Geometry check sheet. Reference: the model listing, model coordinates, mm. A direction names the side the tool comes from. Coordinates: 2 decimals unless noted, no trailing zeros. Loops run counter-clockwise (first coordinate to the right, second up) from the corner with the lowest first, then second, coordinate; pieces in that order, holes last. Notation, with made-up numbers: M 42,22 L 95,22 A24 ccw 95,48 Z; hole C 17,46 d1. An arc over 180 degrees is marked long. One line per question, with ' | ' between items. Start each with the question number.
from build123d import *

# Parameters (mm, degrees)
ESQUISSE1_R             = 12.5
ESQUISSE1_R_2           = 1.25
ESQUISSE1_R_3           = 2.613961031
DISQUE_O25_DEPTH        = 2.5
ESQUISSE2_R             = 5
ESQUISSE2_R_2           = 2.9
MOYEU_CANNELE_25T_DEPTH = 3.5


with BuildPart() as part:
    # Esquisse1 → Disque O25 (new body)
    with BuildSketch(Plane.XY):
        Circle(ESQUISSE1_R)
        with Locations((5, 0)):
            Circle(ESQUISSE1_R_2, mode=Mode.SUBTRACT)
        with Locations((-5, 0)):
            Circle(ESQUISSE1_R_2, mode=Mode.SUBTRACT)
        with Locations((5, 6.363961031)):
            Circle(ESQUISSE1_R_3, mode=Mode.SUBTRACT)
        with Locations((5, -6.363961031)):
            Circle(ESQUISSE1_R_3, mode=Mode.SUBTRACT)
    extrude(amount=DISQUE_O25_DEPTH)

    # Esquisse2 → Moyeu cannele 25T (add)
    with BuildSketch(Plane.XY):
        Circle(ESQUISSE2_R)
        Circle(ESQUISSE2_R_2, mode=Mode.SUBTRACT)
    extrude(amount=-MOYEU_CANNELE_25T_DEPTH)


solid = part.part
1. Tool access check on faces 1 (the cylindrical face through (-6.25, 0.05, 1.23)), 2 (the flat face through (0, 0, 0)), 3 (the cylindrical face through (2.39, 6.48, 1.23)). Record the directions out of +Z, -Z, +X, -X, +Y, -Y that give a thin tool (end or side, any length) a straight path to the whole face; none if there is none.
2. Sectioned sample at B-B (y = -5.75). Record the cut outline in (x, z).
3. Thickness scan on line 1 (Y direction, x = 5, z = 1.2); line 2 (Z direction, x = 8, y = 1.25); line 3 (Y direction, x = -1, z = -0.6). Record the ranges inside material, lowest first.
4. Draft check along Y on faces 4 (the cylindrical face through (11.923, 3.755, 1.232)), 5 (the cylindrical face through (2.926, -7.955, 1.232)), 6 (the flat face through (2.2, -2.2, -3.5)). Enter one of: +Y half, -Y half, draft (parallel to the pull), parting line (faces both ways), or undercut.
5. Sectioned sample at D-D (x = 0). Record the cut outline in (y, z), and give its area (3 significant figures).
6. Sectioned sample at A-A (y = 0). Record the cut outline in (x, z).
7. Sectioned sample at C-C (z = -1.55). Record the cut outline in (x, y).
8. Depth check by flat-ended pin: pin 1 Ø4 at (x, y) = (5, -6.36) entering from -Z; pin 2 Ø1 at (y, z) = (5, 1) entering from -X; pin 3 Ø1.7 at (x, y) = (-0.5, 0) entering from -Z; pin 4 Ø0.6 at (x, y) = (-4.5, 0) entering from +Z. Enter the tip coordinate at first touch or a pass-through.
Result:
1) face 1: +Z | face 2: -Z | face 3: +Z, -Z
2) outline: M -11.1,0 L 2.46,0 L 2.46,2.5 L -11.1,2.5 Z; M 7.54,0 L 11.1,0 L 11.1,2.5 L 7.54,2.5 Z
3) line 1: y = -11.46 to -8.98, -3.75 to -1.25, 1.25 to 3.75, 8.98 to 11.46 | line 2: z = 0 to 2.5 | line 3: y = -4.9 to -2.72, 2.72 to 4.9
4) face 4: parting line | face 5: undercut | face 6: draft
5) outline: M -12.5,0 L -5,0 L -5,-3.5 L -2.9,-3.5 L -2.9,0 L 2.9,0 L 2.9,-3.5 L 5,-3.5 L 5,0 L 12.5,0 L 12.5,2.5 L -12.5,2.5 Z | area: 77.2 mm2
6) outline: M -12.5,0 L -6.25,0 L -6.25,2.5 L -12.5,2.5 Z; M -5,-3.5 L -2.9,-3.5 L -2.9,0 L 2.9,0 L 2.9,-3.5 L 5,-3.5 L 5,0 L 3.75,0 L 3.75,2.5 L -3.75,2.5 L -3.75,0 L -5,0 Z; M 6.25,0 L 12.5,0 L 12.5,2.5 L 6.25,2.5 Z
7) outline: C 0,0 d10; hole C 0,0 d5.8
8) pin 1: passes through | pin 2: stops at x = -11.66 | pin 3: stops at z = 0 | pin 4: stops at z = 0
